Can you work these out from the model? Positions are in its coordinate system, mm. A direction names the side the tool comes from. Give positions to 0.01 mm unless a question says otherwise; leave off trailing zeros. Order: outer loops, then holes, each group sorted by start corner. A loop starts at its lowest first (then second) coordinate and runs counter-clockwise, first axis right, second up. Notation, with made-up numbers: (6, 46) - (45, 46) arc R27 ccw to (45, 75) - close; hole circle Ø7 at (11, -18.75). An arc over 180 degrees is marked (long way). Return JSON: item names as keys, results as strings.
```python
from build123d import *

# Parameters (mm, degrees)
EXTRUDE_1_DEPTH = 3
EXTRUDE_START   = 3
SKETCH_2_R      = 1.35
SKETCH_2_R_2    = 3.25
EXTRUDE_2_DEPTH = 4
FILLET_1_R      = 5


with BuildPart() as part:
    # 草圖1 → 填料-伸長1 (new body)
    with BuildSketch(Plane.XY):
        with BuildLine():
            Line((25.7, -30), (25.7, 30))
            ThreePointArc((25.7, 30), (24.030508653, 34.030508653), (20, 35.7))
            Line((20, 35.7), (-20, 35.7))
            ThreePointArc((-20, 35.7), (-24.030508653, 34.030508653), (-25.7, 30))
            Line((-25.7, 30), (-25.7, -30))
            ThreePointArc((-25.7, -30), (-24.030508653, -34.030508653), (-20, -35.7))
            Line((-20, -35.7), (20, -35.7))
            ThreePointArc((20, -35.7), (24.030508653, -34.030508653), (25.7, -30))
        make_face()
    extrude(amount=EXTRUDE_1_DEPTH)

    # 草圖2 → 填料-伸長2 (add)
    with BuildSketch(Plane.XY.offset(EXTRUDE_START)):
        with BuildLine():
            Line((30, -30), (30, 30))
            ThreePointArc((30, 30), (27.071067812, 37.071067812), (20, 40))
            Line((20, 40), (-20, 40))
            ThreePointArc((-20, 40), (-27.071067812, 37.071067812), (-30, 30))
            Line((-30, 30), (-30, -30))
            ThreePointArc((-30, -30), (-27.071067812, -37.071067812), (-20, -40))
            Line((-20, -40), (20, -40))
            ThreePointArc((20, -40), (27.071067812, -37.071067812), (30, -30))
        make_face()
        with Locations((0, 38)):
            Circle(SKETCH_2_R, mode=Mode.SUBTRACT)
        with Locations((0, -38)):
            Circle(SKETCH_2_R, mode=Mode.SUBTRACT)
        Circle(SKETCH_2_R_2, mode=Mode.SUBTRACT)
        with Locations((14, -14)):
            Circle(SKETCH_2_R_2, mode=Mode.SUBTRACT)
        with Locations((14, 14)):
            Circle(SKETCH_2_R_2, mode=Mode.SUBTRACT)
    extrude(amount=EXTRUDE_2_DEPTH)

    # 圓角1
    # the kernel refuses this fillet: 5 mm, written as the material it takes off along each edge
    with BuildSketch(Plane(origin=(20, -30, 7), x_dir=(0, -1, 0), z_dir=(-1, 0, 0))) as fillet_1_piece_1:
        with BuildLine():
            CenterArc((5.101020514, -5), FILLET_1_R, 11.536959033, 78.463040967)
            Line((5.101020514, 0), (5.101020514, 0.1))
            Line((5.101020514, 0.1), (10, 0.1))
            Line((10, 0.1), (10.1, 0))
            ThreePointArc((10.1, 0), (10.1, -2), (10.09797959, -3.98))
            Line((10.09797959, -3.98), (10, -4))
        make_face()
    revolve(axis=Axis((20, -30, 7), (0, 0, 1)), revolution_arc=90, mode=Mode.SUBTRACT)
    with BuildSketch(Plane(origin=(30, -30, 7), x_dir=(-1.5640821970914211e-12, 0, -1.0), z_dir=(0, 1, 0)), Plane(origin=(-30, 30, 7), x_dir=(1.5640821970914211e-12, 0, -1.0), z_dir=(0, -1, 0))) as fillet_1_piece_2:
        with BuildLine():
            CenterArc((5, 4.898979486), FILLET_1_R, 180, 78.463040967)
            Line((0, 4.898979486), (-0.1, 4.898979486))
            Line((-0.1, 4.898979486), (-0.1, 0))
            Line((-0.1, 0), (0, -0.1))
            ThreePointArc((0, -0.1), (2, -0.1), (3.98, -0.09797959))
            Line((3.98, -0.09797959), (4, 0))
        make_face()
    extrude(amount=60, mode=Mode.SUBTRACT)
    with BuildSketch(Plane(origin=(20, 30, 7), x_dir=(1, 0, 0), z_dir=(0, -1, 0))) as fillet_1_piece_3:
        with BuildLine():
            CenterArc((5.101020514, -5), FILLET_1_R, 11.536959033, 78.463040967)
            Line((5.101020514, 0), (5.101020514, 0.1))
            Line((5.101020514, 0.1), (10, 0.1))
            Line((10, 0.1), (10.1, 0))
            ThreePointArc((10.1, 0), (10.1, -2), (10.09797959, -3.98))
            Line((10.09797959, -3.98), (10, -4))
        make_face()
    revolve(axis=Axis((20, 30, 7), (0, 0, 1)), revolution_arc=90, mode=Mode.SUBTRACT)
    with BuildSketch(Plane(origin=(20, 40, 7), x_dir=(0, -1.5667467323505197e-12, -1.0), z_dir=(-1, 0, 0)), Plane(origin=(-20, -40, 7), x_dir=(0, 1.5667467323505197e-12, -1.0), z_dir=(1, 0, 0))) as fillet_1_piece_4:
        with BuildLine():
            CenterArc((5, 4.898979486), FILLET_1_R, 180, 78.463040967)
            Line((0, 4.898979486), (-0.1, 4.898979486))
            Line((-0.1, 4.898979486), (-0.1, 0))
            Line((-0.1, 0), (0, -0.1))
            ThreePointArc((0, -0.1), (2, -0.1), (3.98, -0.09797959))
            Line((3.98, -0.09797959), (4, 0))
        make_face()
    extrude(amount=40, mode=Mode.SUBTRACT)
    with BuildSketch(Plane(origin=(-20, 30, 7), x_dir=(0, 1, 0), z_dir=(1, 0, 0))) as fillet_1_piece_5:
        with BuildLine():
            CenterArc((5.101020514, -5), FILLET_1_R, 11.536959033, 78.463040967)
            Line((5.101020514, 0), (5.101020514, 0.1))
            Line((5.101020514, 0.1), (10, 0.1))
            Line((10, 0.1), (10.1, 0))
            ThreePointArc((10.1, 0), (10.1, -2), (10.09797959, -3.98))
            Line((10.09797959, -3.98), (10, -4))
        make_face()
    revolve(axis=Axis((-20, 30, 7), (0, 0, 1)), revolution_arc=90, mode=Mode.SUBTRACT)
    with BuildSketch(Plane(origin=(-20, -30, 7), x_dir=(-1, 0, 0), z_dir=(0, 1, 0))) as fillet_1_piece_6:
        with BuildLine():
            CenterArc((5.101020514, -5), FILLET_1_R, 11.536959033, 78.463040967)
            Line((5.101020514, 0), (5.101020514, 0.1))
            Line((5.101020514, 0.1), (10, 0.1))
            Line((10, 0.1), (10.1, 0))
            ThreePointArc((10.1, 0), (10.1, -2), (10.09797959, -3.98))
            Line((10.09797959, -3.98), (10, -4))
        make_face()
    revolve(axis=Axis((-20, -30, 7), (0, 0, 1)), revolution_arc=90, mode=Mode.SUBTRACT)


solid = part.part
```
1. Suppose I cut it at D-D (x = 14). List the corners of the cut face in (y, z) for me, plus the area to 3 significant figures.
Checks:
{"outline": "(-40, 3) - (-35.7, 3) - (-35.7, 0) - (35.7, 0) - (35.7, 3) - (40, 3) arc R5 ccw to (35.1, 7) - (17.25, 7) - (17.25, 3) - (10.75, 3) - (10.75, 7) - (-10.75, 7) - (-10.75, 3) - (-17.25, 3) - (-17.25, 7) - (-35.1, 7) arc R5 ccw to start", "area": "472 mm^2"}
2. On a 3-axis mill with a long thin cutter (end or side, diameter ignored), from which of +Z, -Z, +X, -X, +Y, -Y can I reach the whole of each face in a straight line? I mean faces 1 (the face through (25.7, 0, 1)), 2 (the face through (-23.99, 34.07, 1.48)), 3 (the face through (-24.07, -33.99, 1.48)), 4 (the face through (0, 0, 3)), 5 (the face through (0, -35.7, 1)). Say none if no direction works.
Checks:
{"face 1": "-Z, +X, +Y, -Y", "face 2": "-Z, -X, +Y", "face 3": "-Z, -X, -Y", "face 4": "+Z", "face 5": "-Z, +X, -X, -Y"}
3. Suppose I cut it at C-C (z = 1). List the corners of the cut face in (x, y) for me.
Checks:
{"outline": "(-25.7, -30) arc R5.7 ccw to (-20, -35.7) - (20, -35.7) arc R5.7 ccw to (25.7, -30) - (25.7, 30) arc R5.7 ccw to (20, 35.7) - (-20, 35.7) arc R5.7 ccw to (-25.7, 30) - close"}
4. Suppose I cut it at A-A (y = -27). List the corners of the cut face in (x, z) for me, plus the area to 3 significant figures.
Checks:
{"outline": "(-30, 3) - (-25.7, 3) - (-25.7, 0) - (25.7, 0) - (25.7, 3) - (30, 3) arc R5 ccw to (25.1, 7) - (-25.1, 7) arc R5 ccw to start", "area": "384 mm^2"}
5. Thinking about a two-plate mould opening in X: for faces 6 (the face through (-25.7, 0, 1)), 7 (the face through (14, 14, 3)), 8 (the face through (-6, 0, 7)), which applies, +X half, -X half, draft (parallel to the pull), parting line (faces both ways), or undercut?
Checks:
{"face 6": "-X half", "face 7": "undercut", "face 8": "draft"}
6. Suppose I cut it at B-B (x = 0). List the corners of the cut face in (y, z) for me.
Checks:
{"outline": "(-40, 3) - (-39.35, 3) - (-39.35, 4.64) arc R5 ccw to start; (-36.65, 3) - (-35.7, 3) - (-35.7, 0) - (35.7, 0) - (35.7, 3) - (36.65, 3) - (36.65, 6.75) arc R5 ccw to (35.1, 7) - (3.25, 7) - (3.25, 3) - (-3.25, 3) - (-3.25, 7) - (-35.1, 7) arc R5 ccw to (-36.65, 6.75) - close; (39.35, 3) - (40, 3) arc R5 ccw to (39.35, 4.64) - close"}
7. For pin 1 Ø2 at (y, z) = (24.5, 5.5) entering from -X; pin 2 Ø3 at (x, y) = (13.5, -14) entering from +Z; pin 3 Ø4.5 at (x, y) = (0, -38) entering from +Z, each with a flat end and sliding along its axis, tell me the tip position at first contact or that it passes through.
Checks:
{"pin 1": "x = -29.43", "pin 2": "z = 3", "pin 3": "z = 6.96"}
8. If I drill on L1, parallel to Y at x = 0, z = 4.1; L2, parallel to Y at x = 0, z = 5.2; L3, parallel to Y at x = 2, z = 2.5, over which ranges is the centre line in solid material (lowest first)? Write a range as [from, to].
Checks:
{"L1": "[-39.64, -39.35], [-36.65, -3.25], [3.25, 36.65], [39.35, 39.64]", "L2": "[-36.65, -3.25], [3.25, 36.65]", "L3": "[-35.7, 35.7]"}
